CAD build for the part. Positions are in the model's coordinates, mm. A direction names the side the tool comes from. Give positions to 0.01 mm unless a question says otherwise; leave off trailing zeros. Loops run counter-clockwise (first coordinate to the right, second up) from the corner with the lowest first, then second, coordinate; pieces in that order, holes last.
Item 1: Mould opens along X. For faces 3 (the flat face through (11.96, 1, 106)), 4 (the flat face through (8.785, 1, 106)), 5 (the flat face through (-1, 13.678, 106)) say: released by +X, released by -X, zero draft, split by the parting line, or undercut.
Item 2: Saw through at B-B on z = 184. Give the cut face in (x, y) (3 decimals), plus the area to 3 significant figures.
Item 3: Saw through at A-A on y = 2.25. Give the cut face in (x, z) (3 decimals).
Item 4: Drop a flat-ended pin along its axis: P1, Ø6, axis at x = 5, y = -6.5, coming from the +Z side. Give the stop position or say it passes through.
Item 5: Saw through at C-C on x = -3.25. Give the cut face in (y, z), plus the area to 3 significant figures.
Item 6: Probe probe 1 along X at (y, z) = (6.25, 89.5); probe 2 along Y at (x, z) = (2.75, 203); probe 3 along X at (y, z) = (10.75, 82.5). List the from-to ranges inside material, lowest first.
Item 7: Which spindle directions (+Z, -Z, +X, -X, +Y, -Y) get a long thin tool onto all of the face, cutting with end or side? Do faces 1 (the flat face through (-0.56, -10.49, 12.52)), 2 (the flat face through (-10.265, 1, 107)). Say none if no direction does.
from build123d import *

# Parameters (mm, degrees)
F1_DEPTH = 215.5261469047
F4_DEPTH = 25.4
F5_DEPTH = 25.4


with BuildPart() as f1:
    # F0 (on Top) → F1 (new body)
    with BuildSketch(Plane.XY):
        with BuildLine():
            Line((-10.2649833994, -11.722455886), (8.7850166006, -11.722455886))
            ThreePointArc((8.7850166006, -11.722455886), (11.0300806309, -10.7925199163), (11.9600166006, -8.547455886))
            Line((11.9600166006, -8.547455886), (11.9600166006, 10.502544114))
            ThreePointArc((11.9600166006, 10.502544114), (11.0300806309, 12.7476081443), (8.7850166006, 13.677544114))
            Line((8.7850166006, 13.677544114), (-10.2649833994, 13.677544114))
            ThreePointArc((-10.2649833994, 13.677544114), (-12.5100474297, 12.7476081443), (-13.4399833994, 10.502544114))
            Line((-13.4399833994, 10.502544114), (-13.4399833994, -8.547455886))
            ThreePointArc((-13.4399833994, -8.547455886), (-12.5100474297, -10.7925199163), (-10.2649833994, -11.722455886))
        make_face()
        with BuildLine():
            ThreePointArc((8.7850166006, -5.372455886), (7.8550806309, -7.6175199163), (5.6100166006, -8.547455886))
            Line((5.6100166006, -8.547455886), (-7.0899833994, -8.547455886))
            ThreePointArc((-7.0899833994, -8.547455886), (-9.3350474297, -7.6175199163), (-10.2649833994, -5.372455886))
            Line((-10.2649833994, -5.372455886), (-10.2649833994, 7.327544114))
            ThreePointArc((-10.2649833994, 7.327544114), (-9.3350474297, 9.5726081443), (-7.0899833994, 10.502544114))
            Line((-7.0899833994, 10.502544114), (5.6100166006, 10.502544114))
            ThreePointArc((5.6100166006, 10.502544114), (7.8550806309, 9.5726081443), (8.7850166006, 7.327544114))
            Line((8.7850166006, 7.327544114), (8.7850166006, -5.372455886))
        make_face(mode=Mode.SUBTRACT)
    extrude(amount=F1_DEPTH)

    # F2 (on Front) → F4 (cut, symmetric)
    with BuildSketch(Plane.XZ):
        Polygon((-13.4399833994, 0), (11.9600166006, 0), (-13.4399833994, 25.4), align=None)
    extrude(amount=F4_DEPTH, both=True, mode=Mode.SUBTRACT)

    # F3 (on Front) → F5 (cut, symmetric)
    with BuildSketch(Plane.XZ):
        Polygon((-13.4399833994, 215.5261469047), (-13.4399833994, 190.1261469047), (11.9600166006, 215.5261469047), align=None)
    extrude(amount=F5_DEPTH, both=True, mode=Mode.SUBTRACT)


solid = f1.part
Results below:
1. face 3: released by +X
1. face 4: undercut
1. face 5: zero draft
2. outline: (-13.44, -8.547) arc R3.175 ccw to (-10.265, -11.722) - (8.785, -11.722) arc R3.175 ccw to (11.96, -8.547) - (11.96, 10.503) arc R3.175 ccw to (8.785, 13.678) - (-10.265, 13.678) arc R3.175 ccw to (-13.44, 10.503) - close; hole (-10.265, -5.372) arc R3.175 ccw to (-7.09, -8.547) - (5.61, -8.547) arc R3.175 ccw to (8.785, -5.372) - (8.785, 7.328) arc R3.175 ccw to (5.61, 10.503) - (-7.09, 10.503) arc R3.175 ccw to (-10.265, 7.328) - close
2. area: 282 mm2
3. outline: (-13.44, 25.4) - (-10.265, 22.225) - (-10.265, 193.301) - (-13.44, 190.126) - close; (8.785, 3.175) - (11.96, 0) - (11.96, 215.526) - (8.785, 212.351) - close
4. P1: stops at z = 211.3
5. outline: (-11.72, 15.21) - (-8.55, 15.21) - (-8.55, 200.32) - (-11.72, 200.32) - close; (10.5, 15.21) - (13.68, 15.21) - (13.68, 200.32) - (10.5, 200.32) - close
5. area: 1,180 mm2
6. probe 1: x = -13.44 to -10.26, 8.79 to 11.96
6. probe 2: y = -11.72 to -8.55, 10.5 to 13.68
6. probe 3: x = -13.43 to 11.95
7. face 1: -Z, -X, +Y, -Y
7. face 2: +Z, -Z
